Autodesk Inventor part; units mm, degrees
ref_plane "YZ Plane" through (0, 0, 0) normal (1, 0, 0) x (0, 1, 0)
ref_plane "XZ Plane" through (0, 0, 0) normal (0, 1, 0) x (-1, 0, 0)
ref_plane "XY Plane" through (0, 0, 0) normal (0, 0, 1) x (1, 0, 0)
sketch "Sketch1" plane through (0, 0, 0) normal (1, 0, 0) x (0, 1, 0)
  point P0 (0, 0)
sketch "Sketch2" plane through (0, 0, 0) normal (1, 0, 0) x (0, 1, 0)
  line L0 (29.0822, 42.9634) -> (29.0822, 36.776)
  line L1 (29.0822, 36.776) -> (-3.4283, 11.376)
  line L2 (-3.4283, 11.376) -> (-9.7783, 11.376)
  line L3 (-9.7783, 11.376) -> (-9.7783, 29.8843)
  line L4 (-9.7783, 29.8843) -> (13.0817, 38.4937)
  line L5 (10.2262, 44.396) -> (-9.7798, 44.396)
  line L6 (-9.7798, 44.396) -> (-9.7798, 49.476)
  line L7 (-9.7798, 49.476) -> (29.0822, 49.476)
  line L8 (29.0822, 49.476) -> (29.0822, 42.9634)
  line L9 (10.2262, 44.396) -> (11.4561, 44.396)
  arc A0 (13.0817, 38.4937) -> (11.4561, 44.396) centre (11.4561, 41.221) ccw
  point P0 (0, 0)
  dimension "d0" = 5.08
  dimension "d1" = 6.35
  dimension "d2" = 38.1
  dimension "d3" = 38
  dimension "d4" = 3.175
  dimension "d5" = 21.2344
  dimension "d6" = 12.7
  dimension "d7" = 38.862
  dimension "d9" = 22.86
extrude "Extrusion1" add sketch "Sketch2" along normal blind 12.7
sketch "Sketch4" plane through (0, -9.7798, 49.476) normal (0, 0, 1) x (1, 0, 0)
  point P0 (0, 9.7798)
  point P1 (6.35, 35.3841)
hole "Hole1" at (6.35, 25.6044, 49.476) direction (0, 0, -1) diameter 6.4008 depth 7.62 tip angle 118
sketch "Sketch5" plane through (0, -9.7798, 49.476) normal (0, 0, 1) x (1, 0, 0)
  point P0 (0, 9.7798)
  point P1 (6.35, 2.5513)
hole "Hole2" at (6.35, -7.2284, 49.476) direction (0, 0, -1) diameter 2.54 depth 4.445 tip angle 118
sketch "Sketch6" plane through (12.7, 29.0822, 36.776) normal (0, 0.6157, -0.788) x (-1, 0, 0)
  line L0 (12.7, -46.2603) -> (0, -46.2603) construction
  line L1 (6.35, -46.2603) -> (6.35, -0.205) construction
  line L2 (12.7, 0) -> (0, 0) construction
  point P0 (12.7, -45.5586)
  point P1 (6.35, -8.5344)
  point P2 (6.35, -18.6944)
  point P3 (6.35, -30.1244)
  point P4 (6.35, -38.1)
  dimension "d26" = 8.5344
  dimension "d27" = 18.6944
  dimension "d28" = 30.1244
  dimension "d29" = 38.1
hole "Hole3" at (6.35, 22.357, 31.5217) at (6.35, 14.3508, 25.2665) at (6.35, 5.3439, 18.2295) at (6.35, -0.941, 13.3193) direction (0, -0.6157, 0.788) diameter 5.7404 depth 10.16 tip angle 118
properties part number "Hole part"
Here's how the part is built. I have some questions about the finished solid (model axes, mm). A direction names the side the tool comes from. Round coordinates to 2 decimals unless told otherwise and drop trailing zeros. Order: outer loops, then holes, each group sorted by start corner. A loop starts at its lowest first (then second) coordinate and runs counter-clockwise, first axis right, second up. Notation, with made-up numbers: (32.25, -37.75) -> (47.25, -37.75) arc R24 cw to (47.25, -16.75) -> close; hole circle Ø2 at (-27.5, 56.5). An arc over 180 degrees is marked (long way). Use CSV: the item, a comma, the result in double quotes.
1. I need wall thicknesses on line 1 along Y through (x, z) = (6.35, 47.5); line 2 along Z through (x, y) = (5.75, -4.5); line 3 along Z through (x, y) = (5.5, -5.5). Which ranges of each line are inside material? Lowest first, please.
Recorded:
line 1,"y = -9.78 to -8.5, -5.96 to 22.4, 28.8 to 29.08"
line 2,"z = 11.38 to 13.32, 22.43 to 31.87, 44.4 to 49.48"
line 3,"z = 11.38 to 14.7, 22.95 to 31.5, 44.4 to 49.48"
2. I want a section at B-B on y = -4. Give the number of separate pieces and of enclosed holes in the cut face, and give its area (3 significant figures).
Recorded:
separate pieces,"2"
enclosed holes,"1"
area,"285 mm2"
3. Thinking about a two-plate mould opening in Z: for faces 5 (the face through (6, -7, 11.376)), 6 (the face through (6, -9.778, 21)), 7 (the face through (3.504, 10.885, 29.096)), which applies, pulls with the +Z half, pulls with the -Z half, needs draft (parallel to the pull), parting line crosses it, or undercut?
Recorded:
face 5,"pulls with the -Z half"
face 6,"needs draft"
face 7,"undercut"
4. I want a section at A-A on x = 12. List the corners of the cut face in (y, z) for me (3 decimals).
Recorded:
outline,"(-9.78, 44.396) -> (11.456, 44.396) arc R3.175 cw to (13.082, 38.494) -> (-9.778, 29.884) -> (-9.778, 11.376) -> (-3.428, 11.376) -> (29.082, 36.776) -> (29.082, 49.476) -> (-9.78, 49.476) -> close"
5. Which directions (+Z, -Z, +X, -X, +Y, -Y) give clear straight access to the entire face, cutting with the end or side of a thin tool? Please do faces 1 (the face through (6.047, 6.907, 34.152)), 2 (the face through (6, 29.082, 43)), 3 (the face through (6.26, 1.49, 34.13)), 4 (the face through (8.3, 28.14, 45.61)).
Recorded:
face 1,"none"
face 2,"+Z, -Z, +X, -X, +Y"
face 3,"+X, -X, -Y"
face 4,"+Z"
6. I want a section at C-C on z = 43. List the corners of the cut face in (x, y) for me.
Recorded:
outline,"(0, 14.09) -> (12.7, 14.09) -> (12.7, 29.08) -> (0, 29.08) -> close; hole circle Ø6.4 at (6.35, 25.6)"
7. I'm going to push flat-ended pins straight in: P1, Ø5, axis at x = 6.35, y = 25.6, coming from the +Z side; P2, Ø3, axis at x = 2, z = 22.5, coming from the +Y side. Where does each tip first touch, or does it pass through?
Recorded:
P1,"stops at z = 41.44"
P2,"stops at y = 12.73"
